```python
from build123d import *

# Parameters (mm, degrees)
F0_W     = 200.66
F0_H     = 133.35
F1_DEPTH = 2.54
F2_R     = 5.08
F3_W     = 175.26
F3_H     = 107.95
F4_DEPTH = 5.08
F5_R     = 5.08


with BuildPart() as f1:
    # F0 (on Top) → F1 (new body)
    with BuildSketch(Plane.XY):
        with Locations((-30.6939995439, 1.6928559164)):
            Rectangle(F0_W, F0_H)
    extrude(amount=F1_DEPTH)

    # F2
    f2_edges = [f1.edges().sort_by_distance(p)[0] for p in [
        (69.636, -64.982144, 1.27),
        (69.636, 68.367856, 1.27),
        (-131.024, -64.982144, 1.27),
        (-131.024, 68.367856, 1.27),
    ]]
    fillet(f2_edges, radius=F2_R)

    # F3 (on face) → F4 (cut)
    with BuildSketch(Plane.XY.offset(2.54)):
        with Locations((-30.6939995439, 1.6928559164)):
            Rectangle(F3_W, F3_H)
    extrude(amount=-F4_DEPTH, mode=Mode.SUBTRACT)

    # F5
    f5_edges = [f1.edges().sort_by_distance(p)[0] for p in [
        (-118.324, -52.282144, 1.27),
        (56.936, -52.282144, 1.27),
        (56.936, 55.667856, 1.27),
        (-118.324, 55.667856, 1.27),
    ]]
    fillet(f5_edges, radius=F5_R)


solid = f1.part
```
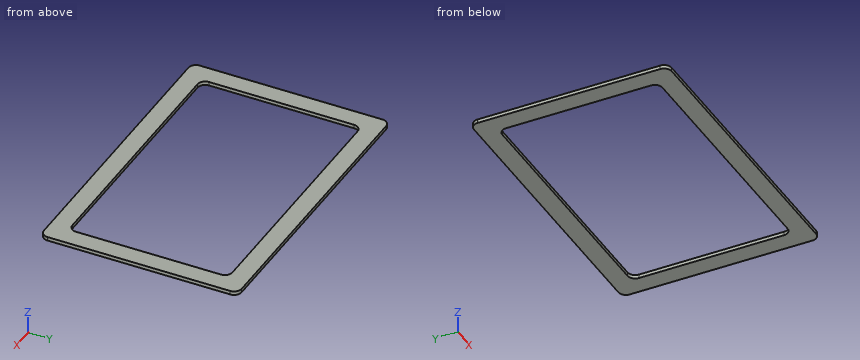
Input: part model. Units: mm. Frame: model coordinates. Coordinates: 2 decimals unless noted, no trailing zeros. Order: outer loops, then holes, each group sorted by start corner. A loop starts at its lowest first (then second) coordinate and runs counter-clockwise, first axis right, second up. Notation, with made-up numbers: (64.5, 74.5) - (84.5, 74.5) arc R22 cw to (84.5, 105.5) - close; hole circle Ø9 at (72.5, 85). An arc over 180 degrees is marked (long way). Put each result on its own line as item: value.
1. Cut plane A-A on z = 1.75. Return the cut outline in (x, y).
Report:
outline: (-131.02, -59.9) arc R5.08 ccw to (-125.94, -64.98) - (64.56, -64.98) arc R5.08 ccw to (69.64, -59.9) - (69.64, 63.29) arc R5.08 ccw to (64.56, 68.37) - (-125.94, 68.37) arc R5.08 ccw to (-131.02, 63.29) - close; hole (-118.32, -47.2) arc R5.08 ccw to (-113.24, -52.28) - (51.86, -52.28) arc R5.08 ccw to (56.94, -47.2) - (56.94, 50.59) arc R5.08 ccw to (51.86, 55.67) - (-113.24, 55.67) arc R5.08 ccw to (-118.32, 50.59) - close
2. Cut plane B-B on x = 22.5. Return the cut outline in (y, z), then the cut area to 3 significant figures.
Report:
outline: (-64.98, 0) - (-52.28, 0) - (-52.28, 2.54) - (-64.98, 2.54) - close; (55.67, 0) - (68.37, 0) - (68.37, 2.54) - (55.67, 2.54) - close
area: 64.5 mm2
3. Cut plane C-C on y = -14.5. Return the cut outline in (x, z).
Report:
outline: (-131.02, 0) - (-118.32, 0) - (-118.32, 2.54) - (-131.02, 2.54) - close; (56.94, 0) - (69.64, 0) - (69.64, 2.54) - (56.94, 2.54) - close
4. Line query: line 1 along Y through (x, z) = (19.5, 1.65); line 2 along X through (y, z) = (15.5, 0.8); line 3 along X through (y, z) = (-51, 2.35). Output: solid intervals per line, ascending.
Report:
line 1: y = -64.98 to -52.28, 55.67 to 68.37
line 2: x = -131.02 to -118.32, 56.94 to 69.64
line 3: x = -131.02 to -116.62, 55.23 to 69.64
